Check sheet for the drawn part. Datum: minimum x, y, z corner. Units: mm. Coordinates: 2 decimals unless noted, no trailing zeros. Write each loop counter-clockwise with the first axis right and the second up, starting at its lowest first coordinate (ties: lowest second). Pieces come first, ordered by that corner, then holes. Notation, with made-up numbers: M 72.5,-24 L 112.5,-24 A23 cw 112.5,15 Z; hole C -4,40 d4. An arc over 180 degrees is marked long. Answer in a Markdown table with one row per item.
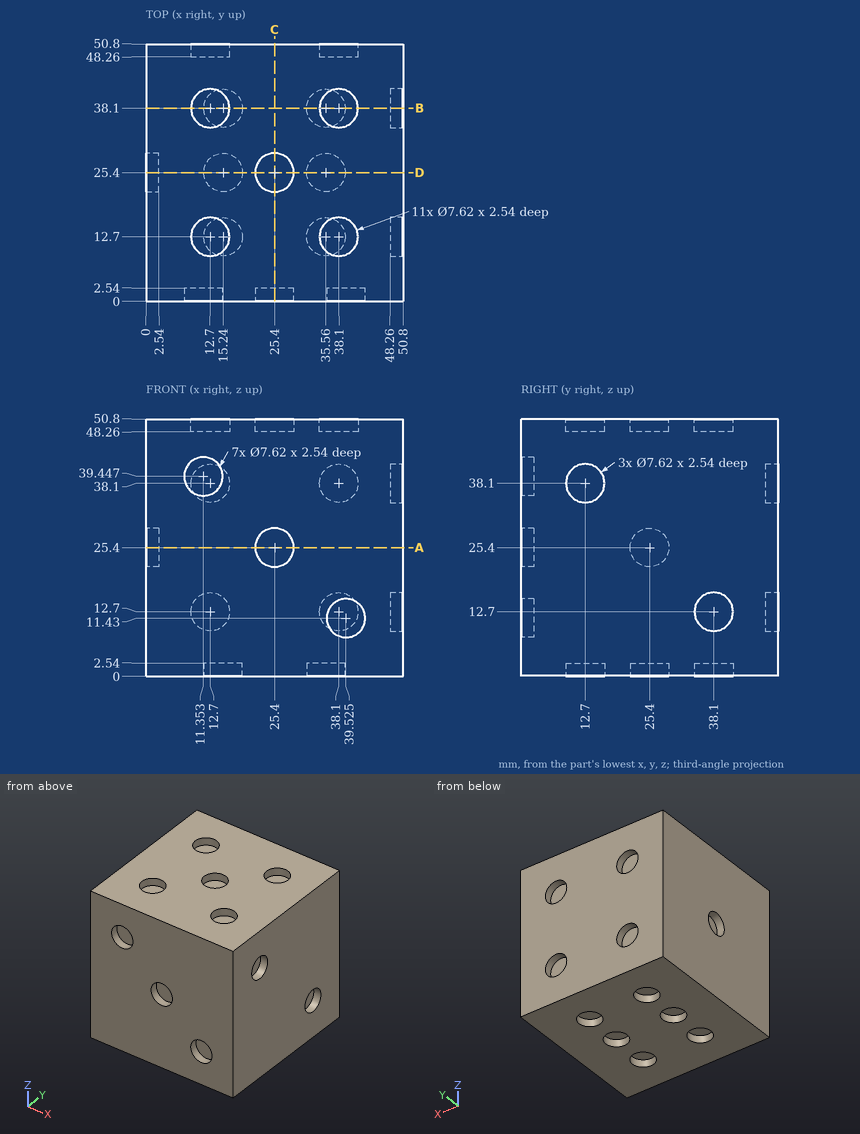
1) Sectioned sample at C-C (x = 25.4). Record the cut outline in (y, z).
Response values:
| item | result |
|---|---|
| outline | M 0,0 L 50.8,0 L 50.8,50.8 L 29.21,50.8 L 29.21,48.26 L 21.59,48.26 L 21.59,50.8 L 0,50.8 L 0,29.21 L 2.54,29.21 L 2.54,21.59 L 0,21.59 Z |
2) Sectioned sample at D-D (y = 25.4). Record the cut outline in (x, z), then the cut area to 3 significant figures.
Response values:
| item | result |
|---|---|
| outline | M 0,0 L 11.43,0 L 11.43,2.54 L 19.05,2.54 L 19.05,0 L 31.75,0 L 31.75,2.54 L 39.37,2.54 L 39.37,0 L 50.8,0 L 50.8,50.8 L 29.21,50.8 L 29.21,48.26 L 21.59,48.26 L 21.59,50.8 L 0,50.8 L 0,29.21 L 2.54,29.21 L 2.54,21.59 L 0,21.59 Z |
| area | 2,500 mm² |
3) Thickness scan on L1, parallel to Y at x = 38.1, z = 49.6; L2, parallel to Z at x = 50, y = 12.7. Record the ranges inside material, lowest first. Write a range as [from, to].
Response values:
| item | result |
|---|---|
| L1 | y = [0, 8.89], [16.51, 34.29], [41.91, 50.8] |
| L2 | z = [0, 34.29], [41.91, 50.8] |
4) Sectioned sample at B-B (y = 38.1). Record the cut outline in (x, z).
Response values:
| item | result |
|---|---|
| outline | M 0,0 L 11.43,0 L 11.43,2.54 L 19.05,2.54 L 19.05,0 L 31.75,0 L 31.75,2.54 L 39.37,2.54 L 39.37,0 L 50.8,0 L 50.8,8.89 L 48.26,8.89 L 48.26,16.51 L 50.8,16.51 L 50.8,50.8 L 41.91,50.8 L 41.91,48.26 L 34.29,48.26 L 34.29,50.8 L 16.51,50.8 L 16.51,48.26 L 8.89,48.26 L 8.89,50.8 L 0,50.8 Z |
5) Depth check by flat-ended pin: pin 1 (7 mm diameter, centred on x = 35.56, y = 12.7, fed in from +Z); pin 2 (6 mm diameter, centred on x = 12.7, y = 12.7, fed in from +Z); pin 3 (2.5 mm diameter, centred on x = 35, y = 23.5, fed in from -Z); pin 4 (6 mm diameter, centred on y = 38.1, z = 12.7, fed in from +X). Enter the tip coordinate at first touch or a pass-through.
Response values:
| item | result |
|---|---|
| pin 1 | stops at z = 50.8 |
| pin 2 | stops at z = 48.26 |
| pin 3 | stops at z = 2.54 |
| pin 4 | stops at x = 48.26 |
6) Sectioned sample at A-A (z = 25.4). Record the cut outline in (x, y), then the cut area to 3 significant figures.
Response values:
| item | result |
|---|---|
| outline | M 0,0 L 21.59,0 L 21.59,2.54 L 29.21,2.54 L 29.21,0 L 50.8,0 L 50.8,50.8 L 0,50.8 L 0,29.21 L 2.54,29.21 L 2.54,21.59 L 0,21.59 Z |
| area | 2,540 mm² |
